Work out the finished part from the listing and answer in its coordinate system (mm). A direction names the side the tool comes from. Give positions to 0.01 mm unless a question says otherwise; leave off trailing zeros. Order: outer loops, then holes, each group sorted by start corner. A loop starts at its lowest first (then second) coordinate and runs counter-clockwise, first axis right, second up. Notation, with made-up numbers: (42, 13.5) -> (61, 13.5) arc R16 ccw to (61, 33.5) -> close; hole circle Ø1 at (40, 2). An arc over 180 degrees is marked (long way). Answer as CSV lines item,"result". Start each with the question number.
1. For a pull along X with two mould halves and no side action, classify faces 3 (the flat face through (694, 1172, -19.05)), 4 (the flat face through (940.333, 172.072, -9.392)), 5 (the flat face through (45.086, 51.32, -9.392)), 6 (the flat face through (945.897, 2067.241, -9.392)) as released by +X, released by -X, zero draft, split by the parting line, or undercut.
2. Find the intervals of material crossed by L1, parallel to Y at x = 348, z = -10; L2, parallel to X at y = 1038, z = -17.75; L3, parallel to Y at x = 510.5, z = -5, in increasing order.
3. A cutting plane is placed at A-A (z = -10.5). Give the vertices of the cut face in (x, y).
4. A cutting plane is placed at C-C (y = 763). Give the vertices of the cut face in (x, z).
5. A cutting plane is placed at D-D (x = 768). Give the vertices of the cut face in (y, z), then the cut area to 3 significant figures.
6. Flat-ended cylindrical pins translate along their axes: pin 1 (4 mm diameter, centred on x = 587, z = -6.5, fed in from +Y) (3 decimals); pin 2 (10 mm diameter, centred on x = 393.5, z = -3, fed in from +Y) (3 decimals); pin 3 (9.5 mm diameter, centred on y = 730.5, z = -13, fed in from -X). Find the tip coordinate at first contact, or state that the pin passes through.
7. For faces 1 (the flat face through (694, 1172, 0)), 2 (the flat face through (946.858, 1407.803, -9.392)), determine the directions among +Z, -Z, +X, -X, +Y, -Y from which every point of the face is accessible in a straight line to the end or side of a thin tool.
8. A cutting plane is placed at B-B (x = 997). Give the vertices of the cut face in (y, z).
from build123d import *

# Parameters (mm, degrees)
F0_W     = 1219.2
F0_H     = 2438.4
F1_DEPTH = 19.05
F3_DEPTH = 25.4
F5_DEPTH = 25.4
F7_DEPTH = 25.4
F9_DEPTH = 25.4


with BuildPart() as f1:
    # F0 (on Top) → F1 (new body)
    with BuildSketch(Plane.XY):
        with Locations((567.030359, 1154.974982)):
            Rectangle(F0_W, F0_H)
    extrude(amount=-F1_DEPTH)

    # F2 (on face) → F3 (cut)
    with BuildSketch(Plane.XY):
        Polygon((414.630359, 1916.974982), (-42.569641, 2374.174982), (-42.569641, 672.374982), (414.630359, 1129.574982), align=None)
    extrude(amount=-F3_DEPTH, mode=Mode.SUBTRACT)

    # F4 (on face) → F5 (cut)
    with BuildSketch(Plane.XY):
        Polygon((414.630359, 1129.574982), (-42.569641, 672.374982), (-42.569641, 138.974982), (135.230359, -38.825018), (414.630359, -38.825018), align=None)
    extrude(amount=-F5_DEPTH, mode=Mode.SUBTRACT)

    # F6 (on face) → F7 (cut)
    with BuildSketch(Plane.XY):
        Polygon((-42.569641, 2374.174982), (414.630359, 1916.974982), (795.630359, 1916.974982), (1100.430359, 2221.774982), (1100.430359, 2374.174982), align=None)
    extrude(amount=-F7_DEPTH, mode=Mode.SUBTRACT)

    # F8 (on face) → F9 (cut)
    with BuildSketch(Plane.XY):
        Polygon((710.56071, 401.844631), (1176.630359, -64.225018), (1176.630359, 1637.574982), (710.56071, 1171.505333), align=None)
    extrude(amount=-F9_DEPTH, mode=Mode.SUBTRACT)


solid = f1.part
Answer sheet:
1,face 3,"zero draft"
1,face 4,"released by +X"
1,face 5,"undercut"
1,face 6,"released by -X"
2,L1,"y = -64.23 to -38.83"
2,L2,"x = 414.63 to 710.56"
2,L3,"y = -64.23 to 1916.97"
3,outline,"(-42.57, -64.23) -> (1176.63, -64.23) -> (710.56, 401.84) -> (710.56, 1171.51) -> (1176.63, 1637.57) -> (1176.63, 2374.17) -> (1100.43, 2374.17) -> (1100.43, 2221.77) -> (795.63, 1916.97) -> (414.63, 1916.97) -> (414.63, -38.83) -> (135.23, -38.83) -> (-42.57, 138.97) -> close"
4,outline,"(414.63, -19.05) -> (710.56, -19.05) -> (710.56, 0) -> (414.63, 0) -> close"
5,outline,"(-64.23, -19.05) -> (344.41, -19.05) -> (344.41, 0) -> (-64.23, 0) -> close; (1228.94, -19.05) -> (1916.97, -19.05) -> (1916.97, 0) -> (1228.94, 0) -> close"
5,area,"20,900 mm^2"
6,pin 1,"stops at y = 1916.975"
6,pin 2,"stops at y = -38.825"
6,pin 3,"stops at x = 414.63"
7,face 1,"+Z, +X, -X, +Y, -Y"
7,face 2,"+Z, -Z, +X"
8,outline,"(-64.23, -19.05) -> (115.41, -19.05) -> (115.41, 0) -> (-64.23, 0) -> close; (1457.94, -19.05) -> (2118.34, -19.05) -> (2118.34, 0) -> (1457.94, 0) -> close"
